Check sheet for the modelled part. Datum: model origin and axes. Units: mm. Face numbers are marked on the shaded views. A direction names the side the tool comes from. Coordinates: 2 decimals unless noted, no trailing zeros. Write each loop counter-clockwise with the first axis right and the second up, starting at its lowest first coordinate (ties: lowest second). Pieces come first, ordered by that corner, then holes. Notation, with made-up numbers: M 39.25,54.25 L 69.25,54.25 A24 ccw 69.25,66.25 Z; hole C 79,-29.75 d1. An arc over 180 degrees is marked long. Answer as CSV lines item,"result". Start each with the question number.
Q1. Sectioned sample at B-B, the plane y = 113. Record the cut outline in (x, z).
Q2. Thickness scan on line 1 along Z through (x, y) = (12.5, 116.25); line 2 along Y through (x, z) = (-29, -141.7); line 3 along Y through (x, z) = (9, -140.05). Record the ranges inside material, lowest first. Write a range as from..to.
Q3. Depth check by flat-ended pin: pin 1 Ø2 at (x, z) = (-42.5, -141.5) entering from +Y; pin 2 Ø1 at (x, z) = (-7.5, -141) entering from +Y; pin 3 Ø1 at (x, z) = (32, -141) entering from -Y; pin 4 Ø4 at (x, y) = (-35.68, 113) entering from -Z. Enter the tip coordinate at first touch or a pass-through.
Q4. Access from +Z, -Z, +X, -X, +Y, -Y to the whole of each face (thin tool, end or side, straight path). Record for the marked faces 1 and 2.
Q5. Sectioned sample at A-A, the plane z = -141.15. Record the cut outline in (x, y).
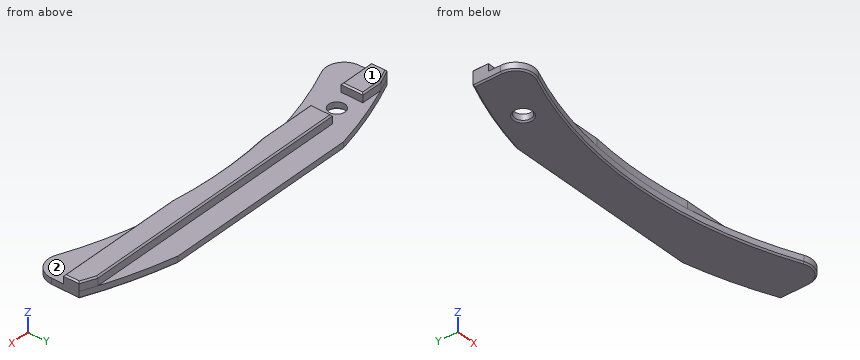
from build123d import *

# Parameters (mm, degrees)
SKETCH290_R     = 2.25
PAD_DEPTH       = 2
PAD074_DEPTH    = 2.4
CHAMFER005_SIZE = 0.4


with BuildPart() as part:
    # Sketch290 → Pad (new body)
    with BuildSketch(Plane.XY):
        with BuildLine():
            Line((-27.221315, 122), (27.221315, 122))
            ThreePointArc((50.682629, 114.264041), (39.143548, 118.713026), (27.221315, 122))
            Line((50.682629, 114.264041), (50.682629, 106.62597))
            ThreePointArc((43.71355, 102.030023), (48.435319, 102.451919), (50.682629, 106.62597))
            ThreePointArc((43.71355, 102.030023), (0, 111), (-43.71355, 102.030023))
            ThreePointArc((-50.682629, 106.62597), (-48.435319, 102.451919), (-43.71355, 102.030023))
            Line((-50.682629, 106.62597), (-50.682629, 114.264041))
            ThreePointArc((-27.221315, 122), (-39.143548, 118.713026), (-50.682629, 114.264041))
        make_face()
        with Locations((-35.682629, 113)):
            Circle(SKETCH290_R, mode=Mode.SUBTRACT)
    extrude(amount=-PAD_DEPTH)

    # Sketch291 → Pad074 (join)
    with BuildSketch(Plane.XY):
        with BuildLine():
            Line((-46.572524, 116), (-40.682629, 116))
            Line((-40.682629, 116), (-40.682629, 110))
            Line((-40.682629, 110), (-50.682629, 110))
            Line((-50.682629, 110), (-50.682629, 114.264041))
            ThreePointArc((-46.572524, 116), (-48.635322, 115.15036), (-50.682629, 114.264041))
        make_face()
        with BuildLine():
            Line((46.572524, 116), (-30.682629, 116))
            Line((-30.682629, 116), (-30.682629, 110))
            Line((-30.682629, 110), (-14.866069, 110))
            ThreePointArc((14.866069, 110), (0, 111), (-14.866069, 110))
            Line((14.866069, 110), (50.682629, 110))
            Line((50.682629, 110), (50.682629, 114.264041))
            ThreePointArc((50.682629, 114.264041), (48.635322, 115.15036), (46.572524, 116))
        make_face()
    extrude(amount=PAD074_DEPTH)

    # Chamfer005
    chamfer005_edges = [part.edges().sort_by_distance(p)[0] for p in [
        (-50.682629, 110.445006, -2),
        (-39.143548, 118.713026, -2),
        (0, 122, -2),
        (39.143548, 118.713026, -2),
        (50.682629, 110.445006, -2),
        (48.435319, 102.451919, -2),
        (0, 111, -2),
        (-48.435319, 102.451919, -2),
        (-37.932629, 113, -2),
        (32.774349, 110, 2.4),
        (50.682629, 112.132021, 2.4),
        (48.635322, 115.15036, 2.4),
        (7.944948, 116, 2.4),
        (-30.682629, 113, 2.4),
        (-22.774349, 110, 2.4),
        (0, 111, 2.4),
        (-43.627576, 116, 2.4),
        (-40.682629, 113, 2.4),
        (-45.682629, 110, 2.4),
        (-50.682629, 112.132021, 2.4),
        (-48.635322, 115.15036, 2.4),
    ]]
    chamfer(chamfer005_edges, length=CHAMFER005_SIZE)


with BuildPart() as part_1:
    # Body022061 placement: moved
    add(part.part.moved(Location((0, 0, -142))))


solid = part_1.part
Output:
1,outline,"M -50.68,-143.6 L -50.28,-144 L -38.33,-144 L -37.93,-143.6 L -37.93,-142 L -40.68,-142 L -40.68,-140 L -41.08,-139.6 L -50.28,-139.6 L -50.68,-140 Z; M -33.43,-143.6 L -33.03,-144 L 50.28,-144 L 50.68,-143.6 L 50.68,-140 L 50.28,-139.6 L -30.28,-139.6 L -30.68,-140 L -30.68,-142 L -33.43,-142 Z"
2,line 1,"z = -144..-142"
2,line 2,"y = 110..116"
2,line 3,"y = 110.63..116"
3,pin 1,"stops at y = 117.86"
3,pin 2,"stops at y = 116"
3,pin 3,"stops at y = 110"
3,pin 4,"passes through"
4,face 1,"+Z, +X, -X, +Y, -Y"
4,face 2,"+Z, +X, -X, -Y"
5,outline,"M -50.68,110 L -40.68,110 L -40.68,116 L -46.57,116 A125 ccw -50.68,114.26 Z; M -30.68,110 L -14.87,110 A111 cw 14.87,110 L 50.68,110 L 50.68,114.26 A125 ccw 46.57,116 L -30.68,116 Z"
